Source: CAD feature listing. Evaluate the final solid. Frame: model axes, mm. Face numbers are marked on the shaded views. Coordinates: 2 decimals unless noted, no trailing zeros. Loops run counter-clockwise (first coordinate to the right, second up) from the corner with the lowest first, then second, coordinate; pieces in that order, holes last. Notation, with made-up numbers: (23.25, 22) -> (64.25, 22) arc R16 cw to (64.25, 36) -> close; hole circle Ø11 at (82, 28.25). An arc over 180 degrees is marked (long way). Answer as a JSON object with one key per item and string values. Group by question number.
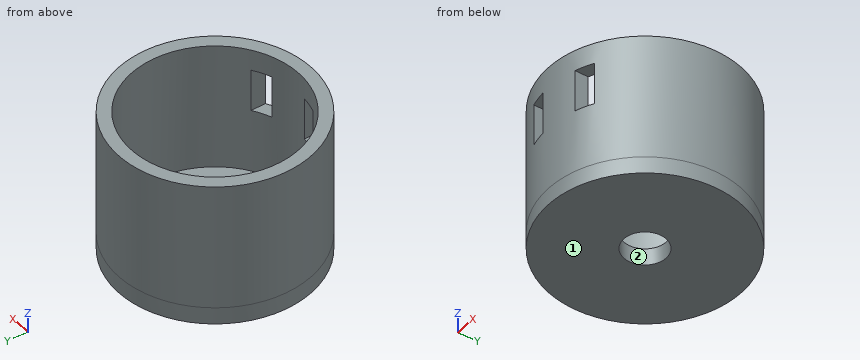
from build123d import *

# Parameters (mm, degrees)
ESQUISSE1_R             = 11.4
ESQUISSE1_R_2           = 9.9
BOSS_EXTRU_1_DEPTH      = 15
BOSS_EXTRU_2_START      = 2
ESQUISSE2_R             = 11.4
ESQUISSE2_R_2           = 2.5
BOSS_EXTRU_2_DEPTH      = 2
ESQUISSE3_W             = 2
ESQUISSE3_H             = 5
ENL_V_MAT_EXTRU_1_DEPTH = 21


with BuildPart() as part:
    # Esquisse1 → Boss.-Extru.1 (new body)
    with BuildSketch(Plane.XY):
        Circle(ESQUISSE1_R)
        Circle(ESQUISSE1_R_2, mode=Mode.SUBTRACT)
    extrude(amount=BOSS_EXTRU_1_DEPTH)

    # Esquisse2 → Boss.-Extru.2 (add)
    with BuildSketch(Plane(origin=(0, 0, 0), x_dir=(-1, 0, 0), z_dir=(0, 0, -1)).offset(BOSS_EXTRU_2_START)):
        Circle(ESQUISSE2_R)
        Circle(ESQUISSE2_R_2, mode=Mode.SUBTRACT)
    extrude(amount=-BOSS_EXTRU_2_DEPTH)

    # Esquisse3 → Enlèv. mat.-Extru.1 (cut)
    with BuildSketch(Plane(origin=(0, 0, 0), x_dir=(1, 0, 0), z_dir=(0, 1, 0))):
        with Locations((4.431290854, -10.002963211)):
            Rectangle(ESQUISSE3_W, ESQUISSE3_H)
        with Locations((-2.078658243, -10.002963211)):
            Rectangle(ESQUISSE3_W, ESQUISSE3_H)
    extrude(amount=-ENL_V_MAT_EXTRU_1_DEPTH, mode=Mode.SUBTRACT)


solid = part.part
1. Ray query, L1, parallel to Y at x = 0, z = 11.5; L2, parallel to Y at x = 0, z = -1.1; L3, parallel to Z at x = 1.75, y = -5.25. Return the intervals inside material, ascending.
2. Section query C-C on z = 14. Return loops of the section in (x, y).
3. Mould query, pull axis Y, two halves, no side actions, for the marked faces 1 and 2. Classes: pulls with the +Y half, pulls with the -Y half, needs draft (parallel to the pull), parting line crosses it, or undercut.
4. Section query D-D on x = 6.5. Return loops of the section in (y, z).
5. Pin query (flat end, axial travel): pin 1 Ø8 at (x, z) = (3.5, 13) entering from -Y; pin 2 Ø6 at (x, y) = (0, 0) entering from +Z; pin 3 Ø0.8 at (y, z) = (-10.5, 9) entering from +X; pin 4 Ø1.4 at (y, z) = (-9, 10.5) entering from -X. Return the tip coordinate at first contact, or that it passes through.
6. Section query A-A on x = 0. Return loops of the section in (y, z), then the cut area to 3 significant figures.
Solved:
{
 "1": {"L1": "-11.4 to -9.9, 9.9 to 11.4", "L2": "-11.4 to -2.5, 2.5 to 11.4", "L3": "-2 to 0"},
 "2": {"outline": "circle Ø22.8 at (0, 0); hole circle Ø19.8 at (0, 0)"},
 "3": {"face 1": "needs draft", "face 2": "undercut"},
 "4": {"outline": "(-9.37, -2) -> (9.37, -2) -> (9.37, 15) -> (7.47, 15) -> (7.47, 0) -> (-7.47, 0) -> (-7.47, 15) -> (-9.37, 15) -> close"},
 "5": {"pin 1": "y = -11.4", "pin 2": "z = 0", "pin 3": "x = 3.43", "pin 4": "x = -7.81"},
 "6": {"outline": "(-11.4, -2) -> (-2.5, -2) -> (-2.5, 0) -> (-9.9, 0) -> (-9.9, 15) -> (-11.4, 15) -> close; (2.5, -2) -> (11.4, -2) -> (11.4, 15) -> (9.9, 15) -> (9.9, 0) -> (2.5, 0) -> close", "area": "80.6 mm^2"}
}
